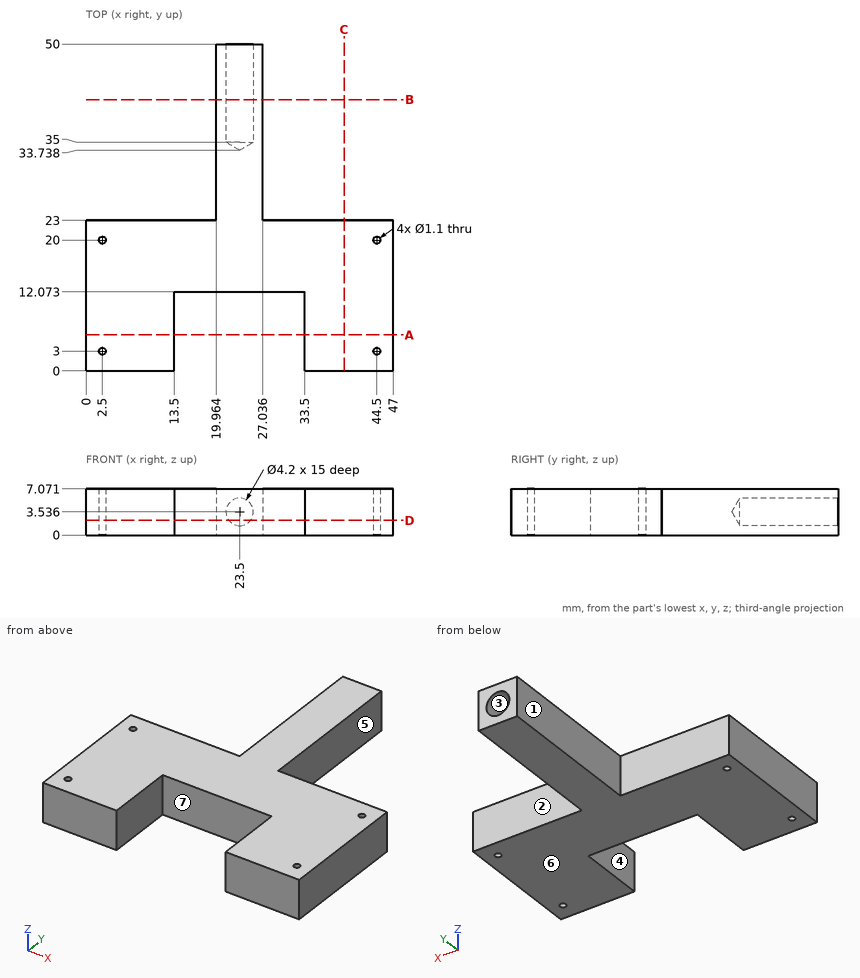
Could you check a few things on this drawing? It's one solid part, dimensions in mm from its lowest x, y, z. A direction names the side the tool comes from. Round coordinates to 2 decimals unless told otherwise and drop trailing zeros. Loops run counter-clockwise (first coordinate to the right, second up) from the corner with the lowest first, then second, coordinate; pieces in that order, holes last. Notation, with made-up numbers: (74.5, -22.5) -> (91.5, -22.5) arc R29 ccw to (91.5, 4.5) -> close; hole circle Ø3 at (7, -28). An arc over 180 degrees is marked (long way). One line per item, written item: value. Start each with the question number.
1. For pin 1 (3.5 mm diameter, centred on x = 7, z = 5, fed in from +Y); pin 2 (5 mm diameter, centred on x = 15.5, y = 40.5, fed in from +Z); pin 3 (4 mm diameter, centred on y = 29, z = 4, fed in from -X); pin 4 (3 mm diameter, centred on x = 26.5, z = 5.5, fed in from -Y), each with a flat end and sliding along its axis, tell me the tip position at first contact or that it passes through.
2. If I drill on probe 1 along Y at (x, z) = (44.5, 4.75); probe 2 along Z at (x, y) = (23.5, 39.5) (1 decimal); probe 3 along X at (y, z) = (4.5, 4.5), over which ranges is the centre line in solid material (lowest first)?
3. If we mould it in two halves opening along X, with no side actions, what happens to the marked faces 5, 6 and 7? For each: pulls with the +X half, pulls with the -X half, needs draft (parallel to the pull), parting line crosses it, or undercut.
4. If we section it at D-D, the plane z = 2.25: Give the number of separate pieces and of enclosed holes in the cut face, then the cut area to 3 significant figures.
5. If we section it at C-C, the plane x = 39.5: Write out the boundary of the cut face in (y, z).
6. For the marked faces 1, 2, 3 and 4, which set-ups out of +Z, -Z, +X, -X, +Y, -Y let a thin tool reach every point of the face, with its end or its side?
7. If we section it at A-A, the plane y = 5.5: Write out the boundary of the cut face in (x, z), then the cut area to 3 significant figures.
8. If we section it at B-B, the plane y = 41.5: Write out the boundary of the cut face in (x, z) (1 decimal).
Calculated:
1. pin 1: stops at y = 23
1. pin 2: passes through
1. pin 3: stops at x = 19.96
1. pin 4: stops at y = 12.07
2. probe 1: y = 0 to 2.45, 3.55 to 19.45, 20.55 to 23
2. probe 2: z = 0 to 1.4, 5.6 to 7.1
2. probe 3: x = 0 to 13.5, 33.5 to 47
3. face 5: pulls with the +X half
3. face 6: needs draft
3. face 7: undercut
4. separate pieces: 1
4. enclosed holes: 4
4. area: 976 mm²
5. outline: (0, 0) -> (23, 0) -> (23, 7.07) -> (0, 7.07) -> close
6. face 1: +Z, -Z, -X, +Y
6. face 2: +Z, -Z, +X, +Y
6. face 3: +Y
6. face 4: +Z, -Z, -Y
7. outline: (0, 0) -> (13.5, 0) -> (13.5, 7.07) -> (0, 7.07) -> close; (33.5, 0) -> (47, 0) -> (47, 7.07) -> (33.5, 7.07) -> close
7. area: 191 mm²
8. outline: (20, 0) -> (27, 0) -> (27, 7.1) -> (20, 7.1) -> close; hole circle Ø4.2 at (23.5, 3.5)
